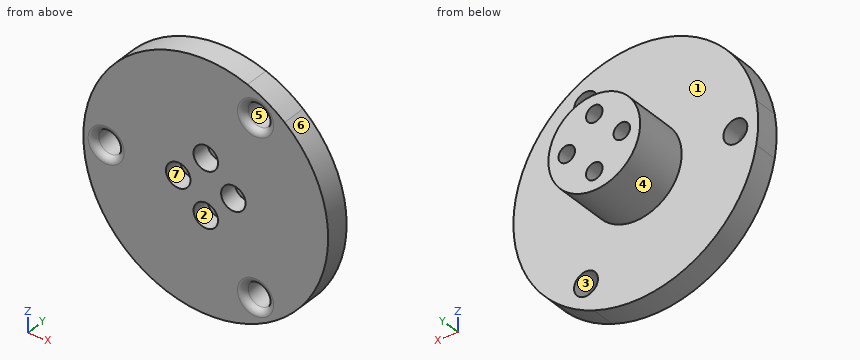
Autodesk Inventor part; units mm, degrees
ref_plane "YZ Plane" through (0, 0, 0) normal (1, 0, 0) x (0, 1, 0)
ref_plane "XZ Plane" through (0, 0, 0) normal (0, 1, 0) x (-1, 0, 0)
ref_plane "XY Plane" through (0, 0, 0) normal (0, 0, 1) x (1, 0, 0)
sketch "Sketch1" plane through (0, 0, 0) normal (0, 1, 0) x (-1, 0, 0)
  circle A0 centre (16.272, 0) radius 1.95
  line L0 (14.741, 3.5) -> (19.6914, 3.5)
  line L1 (14.741, -3.5) -> (19.6914, -3.5)
  line L2 (14.741, 3.5) -> (12, 3.5)
  line L3 (14.741, -3.5) -> (12, -3.5)
  line L4 (-2.9689, 12.1423) -> (-6.8146, 18.8032)
  line L5 (-12.8768, 15.3032) -> (-9.0311, 8.6423)
  line L6 (12, -3.5) -> (19.6914, -3.5)
  line L7 (12, 3.5) -> (19.6914, 3.5)
  line L8 (-2.9689, -12.1423) -> (-6.8146, -18.8032)
  line L9 (-9.0311, -8.6423) -> (-12.8768, -15.3032)
  arc A1 (-6.8146, 18.8032) -> (-12.8768, 15.3032) centre (0, 0) ccw
  arc A2 (-12.8768, -15.3032) -> (-6.8146, -18.8032) centre (0, 0) ccw
  arc A3 (19.6914, -3.5) -> (19.6914, 3.5) centre (0, 0) ccw
  arc A4 (-9.0311, 8.6423) -> (-9.0311, -8.6423) centre (0, 0) ccw
  arc A5 (-2.9689, -12.1423) -> (12, -3.5) centre (0, 0) ccw
  arc A6 (12, 3.5) -> (-2.9689, 12.1423) centre (0, 0) ccw
  line L10 (0, 0) -> (16.272, 0)
  circle A7 centre (-8.136, 14.092) radius 1.95
  circle A8 centre (-8.136, -14.092) radius 1.95
  dimension "d6" = 3.9
  dimension "d20" = 16.272
  dimension "d23" = 360
extrude "Extrusion1" add sketch "Sketch1" along normal blind 4
sketch "Sketch2" plane through (0, 4, 0) normal (0, 1, 0) x (1, 0, 0)
  circle A0 centre (0, 0) radius 7.5
extrude "Extrusion2" add sketch "Sketch2" along normal blind 6
sketch "Sketch3" plane through (0, 10, 0) normal (0, 1, 0) x (1, 0, 0)
  circle A0 centre (-4.5, 0) radius 1.35
  circle A1 centre (0, -4.5) radius 1.35
  circle A2 centre (4.5, 0) radius 1.35
  circle A3 centre (0, 4.5) radius 1.35
  point P0 (0, 0)
  point P1 (0, 0)
  dimension "d26" = 2.7
  dimension "d30" = 360
extrude "Extrusion3" cut sketch "Sketch3" against normal through all
sketch "Sketch4" plane through (0, 0, 0) normal (0, -1, 0) x (1, 0, 0)
  circle A0 centre (-4.5, 0) radius 1.35
  circle A1 centre (-4.5, 0) radius 2
  circle A2 centre (0, -4.5) radius 2
  circle A3 centre (4.5, 0) radius 2
  circle A4 centre (0, 4.5) radius 2
  point P0 (0, 0)
  point P1 (0, 0)
  dimension "d34" = 4
  dimension "d37" = 360
extrude "Extrusion4" cut sketch "Sketch4" against normal blind 3
sketch "Sketch5" plane through (0, 0, 0) normal (0, -1, 0) x (1, 0, 0)
  arc A0 (12.8768, 15.3032) -> (6.8146, 18.8032) centre (0, 0) ccw
  arc A1 (-19.6914, 3.5) -> (-19.6914, -3.5) centre (0, 0) ccw
  line L0 (-19.6914, 3.5) -> (-12, 3.5)
  line L1 (-19.6914, 3.5) -> (-12, 3.5)
  line L2 (-12, -3.5) -> (-19.6914, -3.5)
  line L3 (-19.6914, -3.5) -> (-12, -3.5)
  line L4 (6.8146, -18.8032) -> (2.9689, -12.1423)
  line L5 (6.8146, -18.8032) -> (2.9689, -12.1423)
  line L6 (9.0311, -8.6423) -> (12.8768, -15.3032)
  line L7 (12.8768, -15.3032) -> (9.0311, -8.6423)
  line L8 (12.8768, 15.3032) -> (9.0311, 8.6423)
  arc A2 (9.0311, -8.6423) -> (9.0311, 8.6423) centre (0, 0) ccw
  line L9 (12.8768, 15.3032) -> (9.0311, 8.6423)
  line L10 (2.9689, 12.1423) -> (6.8146, 18.8032)
  line L11 (6.8146, 18.8032) -> (2.9689, 12.1423)
  arc A3 (2.9689, 12.1423) -> (-12, 3.5) centre (0, 0) ccw
  arc A4 (2.9689, 12.1423) -> (-12, 3.5) centre (0, 0) ccw
  arc A5 (6.8146, 18.8032) -> (-19.6914, 3.5) centre (0, 0) ccw
  arc A6 (-19.6914, -3.5) -> (6.8146, -18.8032) centre (0, 0) ccw
  arc A7 (12.8768, -15.3032) -> (12.8768, 15.3032) centre (0, 0) ccw
  arc A8 (-12, -3.5) -> (2.9689, -12.1423) centre (0, 0) ccw
  arc A9 (9.0311, -8.6423) -> (9.0311, 8.6423) centre (0, 0) ccw
extrude "Extrusion5" add sketch "Sketch5" against normal up to surface (4 mm away)
fillet "Fillet1" radius 1 3 edges at (10.086, 0, 14.092) (-14.322, 0, 0) (10.086, 0, -14.092)
sketch "Sketch6" plane through (0, 10, 0) normal (0, 1, 0) x (1, 0, 0)
  circle A0 centre (0, 0) radius 7.5
  circle A1 centre (-4.5, 0) radius 1.35
  circle A2 centre (-4.5, 0) radius 1.35
  circle A3 centre (0, 4.5) radius 1.35
  circle A4 centre (0, 4.5) radius 1.35
  circle A5 centre (4.5, 0) radius 1.35
  circle A6 centre (4.5, 0) radius 1.35
  circle A7 centre (0, -4.5) radius 1.35
  circle A8 centre (0, -4.5) radius 1.35
extrude "Extrusion6" add sketch "Sketch6" along normal blind 3
properties part number "Planet_Gear_Output"
Source: CAD feature listing. Evaluate the final solid. Frame: model axes, mm. Face numbers are marked on the shaded views. A direction names the side the tool comes from. Give positions to 0.01 mm unless a question says otherwise; leave off trailing zeros. Write each loop counter-clockwise with the first axis right and the second up, starting at its lowest first coordinate (ties: lowest second). Pieces come first, ordered by that corner, then holes. Notation, with made-up numbers: M -2.5,11 L 13.5,11 A26 cw 13.5,50 Z; hole C -17,79.25 d6. An arc over 180 degrees is marked long. Return JSON: item names as keys, results as strings. Group by question number.
1) Draft query along X for the marked faces 4, 5, 6 and 7. Return one class per face: released by +X, released by -X, zero draft, split by the parting line, or undercut.
2) Cut plane C-C, the plane y = 2. Output: boundary loops of the cut face in (x, z), then the cut area to 3 significant figures.
3) First-contact query: pin 1 Ø3 at (y, z) = (5, -12.5) entering from +X; pin 2 Ø6 at (x, z) = (8.136, 14.092) entering from -Y; pin 3 Ø2 at (y, z) = (10, -5) entering from -X; pin 4 Ø4 at (x, y) = (4, 3.5) entering from -Z. Flat tips, straight axial feed; report the tip coordinate or a pass-through.
4) Cut plane A-A, the plane z = 0. Give the number of separate pieces and of enclosed holes in the cut face, then the cut area to 3 significant figures.
5) Set-up query: the marked faces 1, 2 and 3. Return all of +Z, -Z, +X, -X, +Y, -Y with unobstructed straight access to the full face (end or side cutting, diameter ignored); none if empty.
6) Cut plane B-B, the plane x = 0. Output: boundary loops of the cut face in (y, z), then the cut area to 3 significant figures.
7) Ray query, L1, parallel to Z at x = 0, y = 5.25; L2, parallel to Y at x = 15.5, z = 10.5. Return the intervals inside material, ascending.
8) Cut plane D-D, the plane z = 4.5. Output: boundary loops of the cut face in (x, y).
Data:
{
 "1": {"face 4": "split by the parting line", "face 5": "undercut", "face 6": "released by +X", "face 7": "undercut"},
 "2": {"outline": "M -19.69,-3.5 A20 ccw 6.81,-18.8 A20 ccw 12.88,-15.3 A20 ccw 12.88,15.3 A20 ccw 6.81,18.8 A20 ccw -19.69,3.5 A20 ccw Z; hole C -16.27,0 d3.9; hole C -4.5,0 d4; hole C 0,-4.5 d4; hole C 0,4.5 d4; hole C 4.5,0 d4; hole C 8.14,-14.09 d3.9; hole C 8.14,14.09 d3.9", "area": "1,170 mm²"},
 "3": {"pin 1": "stops at x = 16.45", "pin 2": "stops at y = 0", "pin 3": "stops at x = -6.34", "pin 4": "stops at z = -19.9"},
 "4": {"separate pieces": "4", "enclosed holes": "0", "area": "201 mm²"},
 "5": {"face 1": "+Y", "face 2": "-Y", "face 3": "+Y, -Y"},
 "6": {"outline": "M 0,-20 L 4,-20 L 4,-7.5 L 13,-7.5 L 13,-5.85 L 3,-5.85 L 3,-6.5 L 0,-6.5 Z; M 0,-2.5 L 3,-2.5 L 3,-3.15 L 13,-3.15 L 13,3.15 L 3,3.15 L 3,2.5 L 0,2.5 Z; M 0,6.5 L 3,6.5 L 3,5.85 L 13,5.85 L 13,7.5 L 4,7.5 L 4,20 L 0,20 Z", "area": "217 mm²"},
 "7": {"L1": "z = -7.5 to -5.85, -3.15 to 3.15, 5.85 to 7.5", "L2": "y = 0 to 4"},
 "8": {"outline": "M -19.49,0 L -2,0 L -2,3 L -1.35,3 L -1.35,13 L -6,13 L -6,4 L -19.49,4 Z; M 1.35,3 L 2,3 L 2,0 L 19.49,0 L 19.49,4 L 6,4 L 6,13 L 1.35,13 Z"}
}
